```python
from build123d import *

# Parameters (mm, degrees)
SKETCH1_W           = 196.85
SKETCH1_H           = 114.3
SKETCH1_R           = 3.175
BOSS_EXTRUDE1_DEPTH = 6.35
CUT_EXTRUDE1_REACH  = 200.247
SKETCH7_W           = 72.25
SKETCH7_H           = 53.975
CUT_EXTRUDE3_DEPTH  = 6.35
CUT_EXTRUDE4_DEPTH  = 6.35
FILLET1_R           = 4.7625
SKETCH10_R          = 2.4892
CUT_EXTRUDE5_DEPTH  = 6.35


with BuildPart() as part:
    # Sketch1 → Boss-Extrude1 (new body)
    with BuildSketch(Plane(origin=(0, 0, 0), x_dir=(1, 0, 0), z_dir=(0, 1, 0))):
        with Locations((91.3, 0)):
            Rectangle(SKETCH1_W, SKETCH1_H)
        with Locations(Location((0, 41.275, 0), (0, 0, 270))):
            Circle(SKETCH1_R, mode=Mode.SUBTRACT)
        with Locations(Location((0, -41.275, 0), (0, 0, 90))):
            Circle(SKETCH1_R, mode=Mode.SUBTRACT)
        with Locations(Location((57.15, 41.275, 0), (0, 0, 270))):
            Circle(SKETCH1_R, mode=Mode.SUBTRACT)
        with Locations(Location((57.15, -41.275, 0), (0, 0, 90))):
            Circle(SKETCH1_R, mode=Mode.SUBTRACT)
    extrude(amount=BOSS_EXTRUDE1_DEPTH)

    # Sketch2 → Cut-Extrude1 (cut, up to next)
    with BuildSketch(Plane(origin=(0, 6.35, 0), x_dir=(1, 0, 0), z_dir=(0, 1, 0)), mode=Mode.PRIVATE) as cut_extrude1_sk1:
        Polygon((-7.125, 0), (-7.125, -31.75), (53.975, -31.75), (53.975, 0), (53.975, 31.75), (-7.125, 31.75), align=None)
    cut_extrude1_tool1 = extrude(cut_extrude1_sk1.sketch, amount=-CUT_EXTRUDE1_REACH, mode=Mode.PRIVATE) & part.part
    add(cut_extrude1_tool1.solids().sort_by_distance((23.425, 6.35, 0))[0], mode=Mode.SUBTRACT)

    # Sketch7 → Cut-Extrude3 (cut)
    with BuildSketch(Plane.XZ):
        with Locations((153.6, 0)):
            Rectangle(SKETCH7_W, SKETCH7_H)
    extrude(amount=-CUT_EXTRUDE3_DEPTH, mode=Mode.SUBTRACT)

    # Sketch9 → Cut-Extrude4 (cut)
    with BuildSketch(Plane(origin=(0, 6.35, 0), x_dir=(1, 0, 0), z_dir=(0, 1, 0))):
        with BuildLine():
            Line((135.875, -36.322), (123.175, -36.322))
            ThreePointArc((123.175, -36.322), (120, -33.147), (123.175, -29.972))
            Line((123.175, -29.972), (135.875, -29.972))
            ThreePointArc((135.875, -29.972), (139.05, -33.147), (135.875, -36.322))
        make_face()
        with BuildLine():
            Line((161.275, -29.972), (173.975, -29.972))
            ThreePointArc((173.975, -29.972), (177.15, -33.147), (173.975, -36.322))
            Line((173.975, -36.322), (161.275, -36.322))
            ThreePointArc((161.275, -36.322), (158.1, -33.147), (161.275, -29.972))
        make_face()
        with BuildLine():
            Line((161.275, 29.972), (173.975, 29.972))
            ThreePointArc((173.975, 29.972), (177.15, 33.147), (173.975, 36.322))
            Line((173.975, 36.322), (161.275, 36.322))
            ThreePointArc((161.275, 36.322), (158.1, 33.147), (161.275, 29.972))
        make_face()
        with BuildLine():
            Line((135.875, 36.322), (123.175, 36.322))
            ThreePointArc((123.175, 36.322), (120, 33.147), (123.175, 29.972))
            Line((123.175, 29.972), (135.875, 29.972))
            ThreePointArc((135.875, 29.972), (139.05, 33.147), (135.875, 36.322))
        make_face()
        with BuildLine():
            Line((82.56875, 0), (82.56875, -25.4))
            ThreePointArc((82.56875, -25.4), (78.6, -29.36875), (74.63125, -25.4))
            Line((74.63125, -25.4), (74.63125, 0))
            ThreePointArc((74.63125, 0), (78.6, 3.96875), (82.56875, 0))
        make_face()
    extrude(amount=-CUT_EXTRUDE4_DEPTH, mode=Mode.SUBTRACT)

    # Fillet1
    fillet1_edges = [part.edges().sort_by_distance(p)[0] for p in [
        (53.975, 3.175, 31.75),
        (53.975, 3.175, -31.75),
        (117.475, 3.175, 26.9875),
        (117.475, 3.175, -26.9875),
    ]]
    fillet(fillet1_edges, radius=FILLET1_R)

    # Sketch10 → Cut-Extrude5 (cut)
    with BuildSketch(Plane(origin=(0, 6.35, 0), x_dir=(1, 0, 0), z_dir=(0, 1, 0))):
        with Locations(Location((107.95, -6.35, 0), (0, 0, 270))):
            Circle(SKETCH10_R)
        with Locations(Location((107.95, 6.35, 0), (0, 0, 270))):
            Circle(SKETCH10_R)
    extrude(amount=-CUT_EXTRUDE5_DEPTH, mode=Mode.SUBTRACT)


solid = part.part
```
The model under review builds one solid part; all positions refer to its coordinate system, in mm. A direction names the side the tool comes from. Round coordinates to 2 decimals unless told otherwise and drop trailing zeros. Loops run counter-clockwise (first coordinate to the right, second up) from the corner with the lowest first, then second, coordinate; pieces in that order, holes last. Notation, with made-up numbers: (19.5, -25) - (37.5, -25) arc R12 cw to (37.5, -16) - close; hole circle Ø10 at (23.25, -7). An arc over 180 degrees is marked (long way). Write each question's results on one line, items separated by ' | '. Start each with the question number.
Q1. Take a section at A-A on x = 0. Give the boundary of the cut face in (y, z).
Q2. Insertion check: P1, Ø7.5, axis at x = 57.15, z = 41.275, coming from the +Y side; P2, Ø3, axis at y = 2.5, z = 13.5, coming from the +X side (3 decimals). Each pin has a flat end and moves straight along its axis. Give the tip position at first contact, or say it passes through.
Q3. Take a section at D-D on z = -6.35. Give the boundary of the cut face in (x, y) (3 decimals), plus the area to 3 significant figures.
Q4. Take a section at B-B on z = 6.35. Give the boundary of the cut face in (x, y) (3 decimals).
Q5. Wall thickness on line 1 along X through (y, z) = (4.25, 6.35) (3 decimals); line 2 along X through (y, z) = (5.5, 3.5) (3 decimals); line 3 along X through (y, z) = (3.75, -6.35) (3 decimals): over which ranges is each line inside the solid? List them lowest first. Write a range as [from, to].
Q6. Tool access review of faces 1 (the flat face through (156, 3, -26.988)), 2 (the cylindrical face through (120, 3.2, 33.2)), 3 (the flat face through (21, 3, 31.75)): name each direction out of +Z, -Z, +X, -X, +Y, -Y from which nothing blocks a thin tool from reaching the whole face with its end or side.
Q7. Take a section at C-C on x = 107.95. Give the boundary of the cut face in (y, z), plus the area to 3 significant figures.
Q8. Draft analysis for pull direction Z (two halves, no side actions). For faces 4 (the cylindrical face through (177.15, 3.22, -33.08)), 5 (the flat face through (-7.125, 3, -44)), 6 (the flat face through (90, 3, 57.15)), state which applies: pulls with the +Z half, pulls with the -Z half, needs draft (parallel to the pull), parting line crosses it, or undercut.
Data:
1) outline: (0, -57.15) - (6.35, -57.15) - (6.35, -44.45) - (0, -44.45) - close; (0, -38.1) - (6.35, -38.1) - (6.35, -31.75) - (0, -31.75) - close; (0, 31.75) - (6.35, 31.75) - (6.35, 38.1) - (0, 38.1) - close; (0, 44.45) - (6.35, 44.45) - (6.35, 57.15) - (0, 57.15) - close
2) P1: stops at y = 6.35 | P2: stops at x = 117.475
3) outline: (53.975, 0) - (105.461, 0) - (105.461, 6.35) - (53.975, 6.35) - close; (110.439, 0) - (117.475, 0) - (117.475, 6.35) - (110.439, 6.35) - close | area: 372 mm²
4) outline: (53.975, 0) - (74.631, 0) - (74.631, 6.35) - (53.975, 6.35) - close; (82.569, 0) - (105.461, 0) - (105.461, 6.35) - (82.569, 6.35) - close; (110.439, 0) - (117.475, 0) - (117.475, 6.35) - (110.439, 6.35) - close
5) line 1: x = [53.975, 74.631], [82.569, 105.461], [110.439, 117.475] | line 2: x = [53.975, 74.631], [82.569, 117.475] | line 3: x = [53.975, 105.461], [110.439, 117.475]
6) face 1: +X, +Y, -Y | face 2: +Y, -Y | face 3: -X, +Y, -Y
7) outline: (0, -57.15) - (6.35, -57.15) - (6.35, -8.84) - (0, -8.84) - close; (0, -3.86) - (6.35, -3.86) - (6.35, 3.86) - (0, 3.86) - close; (0, 8.84) - (6.35, 8.84) - (6.35, 57.15) - (0, 57.15) - close | area: 663 mm²
8) face 4: undercut | face 5: needs draft | face 6: pulls with the +Z half
